Part model, mm, in its own coordinate system. Coordinates: 2 decimals unless noted, no trailing zeros. Loops run counter-clockwise (first coordinate to the right, second up) from the corner with the lowest first, then second, coordinate; pieces in that order, holes last.
```python
from build123d import *

# Parameters (mm, degrees)
F0_W     = 262.38215
F0_H     = 102.365531
F1_DEPTH = 19.05
F3_D     = 25.4
F5_D     = 9.525


with BuildPart() as f1:
    # F0 (on Top) → F1 (new body)
    with BuildSketch(Plane.XY):
        with Locations((131.191075, 51.182765)):
            Rectangle(F0_W, F0_H)
    extrude(amount=F1_DEPTH)

    # F3 (through all)
    with Locations(Plane.XY.offset(19.05)):
        with Locations((116.925366, 53.350501)):
            Hole(F3_D / 2)

    # F5 (through all)
    with Locations(Plane.XY.offset(19.05)):
        with Locations((14.968506, 81.472881), (15.936192, 27.136751), (241.621628, 83.117127), (244.734511, 25.796823)):
            Hole(F5_D / 2)


solid = f1.part
```
Q1. Mould opens along Y. For faces 1 (the cylindrical face through (16.001, 76.824, 9.392)), 2 (the flat face through (129, 102.366, 9)), 3 (the flat face through (129, 63, 19.05)), 4 (the cylindrical face through (104.812, 57.165, 9.392)) say: released by +Y, released by -Y, zero draft, split by the parting line, or undercut.
Q2. Saw through at C-C (y = 56.5). List the corners of the cut face in (x, z), plus the area to 3 significant figures.
Q3. Saw through at A-A (y = 44). List the corners of the cut face in (x, z), plus the area to 3 significant figures.
Q4. Saw through at B-B (z = 5.75). List the corners of the cut face in (x, y) (1 decimal), plus the area to 3 significant figures.
Q5. Probe line 1 (Y direction, x = 245, z = 4.5); line 2 (X direction, y = 79, z = 11.5); line 3 (X direction, y = 30, z = 5.5). List the from-to ranges inside material, lowest first.
Checked values:
1. face 1: undercut
1. face 2: released by +Y
1. face 3: zero draft
1. face 4: undercut
2. outline: (0, 0) - (104.62, 0) - (104.62, 19.05) - (0, 19.05) - close; (129.23, 0) - (262.38, 0) - (262.38, 19.05) - (129.23, 19.05) - close
2. area: 4,530 mm2
3. outline: (0, 0) - (108.33, 0) - (108.33, 19.05) - (0, 19.05) - close; (125.52, 0) - (262.38, 0) - (262.38, 19.05) - (125.52, 19.05) - close
3. area: 4,670 mm2
4. outline: (0, 0) - (262.4, 0) - (262.4, 102.4) - (0, 102.4) - close; hole circle Ø9.5 at (15, 81.5); hole circle Ø9.5 at (15.9, 27.1); hole circle Ø25.4 at (116.9, 53.4); hole circle Ø9.5 at (241.6, 83.1); hole circle Ø9.5 at (244.7, 25.8)
4. area: 26,100 mm2
5. line 1: y = 0 to 21.04, 30.55 to 79.76, 86.47 to 102.37
5. line 2: x = 0 to 10.9, 19.04 to 239.23, 244.02 to 262.38
5. line 3: x = 0 to 12.13, 19.74 to 242.5, 246.97 to 262.38
